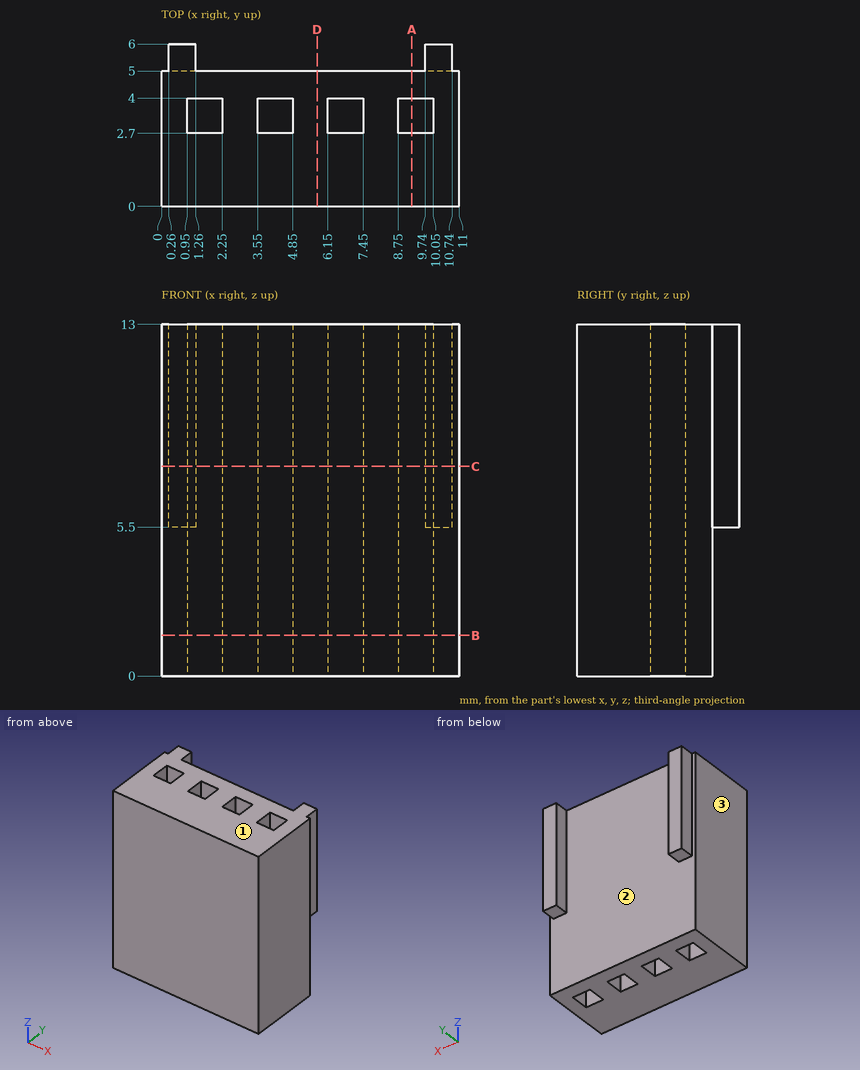
Source: three-view drawing plus pictorial views. Frame: mm from the lowest corner of the part. Round coordinates to 2 decimals unless told otherwise and drop trailing zeros. Loops run counter-clockwise (first coordinate to the right, second up) from the corner with the lowest first, then second, coordinate; pieces in that order, holes last.
1. Section query B-B on z = 1.5. Output: boundary loops of the cut face in (x, y).
2. Section query A-A on x = 9.25. Output: boundary loops of the cut face in (y, z), and give its area (3 significant figures).
3. Ray query, L1, parallel to X at y = 3.4, z = 5.25; L2, parallel to Y at x = 4.75, z = 10.5; L3, parallel to X at y = 5.1, z = 8.5. Return the intervals inside material, ascending.
4. Mould query, pull axis X, two halves, no side actions, for the marked faces 1, 2 and 3. Classes: released by +X, released by -X, zero draft, split by the parting line, or undercut.
5. Section query C-C on z = 7.75. Output: boundary loops of the cut face in (x, y).
6. Section query D-D on x = 5.75. Output: boundary loops of the cut face in (y, z), and give its area (3 significant figures).
7. Contact query for flat-ended pins moving along their axis: pin 1 (1 mm diameter, centred on x = 1.5, z = 9, fed in from +Y); pin 2 (3 mm diameter, centred on x = 6, z = 11.5, fed in from +Y); pin 3 (0.8 mm diameter, centred on y = 5.5, z = 11, fed in from -X). Output: stop coordinate, or through.
Answers below:
1. outline: (0, 0) - (11, 0) - (11, 5) - (0, 5) - close; hole (0.95, 2.7) - (2.25, 2.7) - (2.25, 4) - (0.95, 4) - close; hole (3.55, 2.7) - (4.85, 2.7) - (4.85, 4) - (3.55, 4) - close; hole (6.15, 2.7) - (7.45, 2.7) - (7.45, 4) - (6.15, 4) - close; hole (8.75, 2.7) - (10.05, 2.7) - (10.05, 4) - (8.75, 4) - close
2. outline: (0, 0) - (2.7, 0) - (2.7, 13) - (0, 13) - close; (4, 0) - (5, 0) - (5, 13) - (4, 13) - close
2. area: 48.1 mm2
3. L1: x = 0 to 0.95, 2.25 to 3.55, 4.85 to 6.15, 7.45 to 8.75, 10.05 to 11
3. L2: y = 0 to 2.7, 4 to 5
3. L3: x = 0.26 to 1.26, 9.74 to 10.74
4. face 1: zero draft
4. face 2: undercut
4. face 3: released by -X
5. outline: (0, 0) - (11, 0) - (11, 5) - (10.74, 5) - (10.74, 6) - (9.74, 6) - (9.74, 5) - (1.26, 5) - (1.26, 6) - (0.26, 6) - (0.26, 5) - (0, 5) - close; hole (0.95, 2.7) - (2.25, 2.7) - (2.25, 4) - (0.95, 4) - close; hole (3.55, 2.7) - (4.85, 2.7) - (4.85, 4) - (3.55, 4) - close; hole (6.15, 2.7) - (7.45, 2.7) - (7.45, 4) - (6.15, 4) - close; hole (8.75, 2.7) - (10.05, 2.7) - (10.05, 4) - (8.75, 4) - close
6. outline: (0, 0) - (5, 0) - (5, 13) - (0, 13) - close
6. area: 65.0 mm2
7. pin 1: stops at y = 6
7. pin 2: stops at y = 5
7. pin 3: stops at x = 0.26
